from build123d import *

# Parameters (mm, degrees)
SKETCH_1_W               = 40
SKETCH_1_H               = 29
EXTRUDE_1_DEPTH          = 3
CUT_EXTRUDE_1_DEPTH      = 3
SKETCH_3_W               = 40
SKETCH_3_H               = 3
EXTRUDE_2_DEPTH          = 10
SKETCH_4_W               = 40
SKETCH_4_H               = 3
EXTRUDE_3_DEPTH          = 10
SKETCH_6_W               = 3
SKETCH_6_H               = 49
EXTRUDE_5_DEPTH          = 42
SKETCH_8_W               = 3
SKETCH_8_H               = 49
EXTRUDE_6_DEPTH          = 2
SKETCH_9_W               = 3
SKETCH_9_H               = 49
EXTRUDE_7_DEPTH          = 2
SKETCH_10_W              = 86
SKETCH_10_H              = 3
EXTRUDE_8_DEPTH          = 10
SKETCH_11_W              = 86
SKETCH_11_H              = 3
EXTRUDE_9_DEPTH          = 10
SKETCH_14_W              = 3
SKETCH_14_H              = 69
CUT_EXTRUDE_5_DEPTH      = 43
SKETCH_17_W              = 43
SKETCH_17_H              = 3
EXTRUDE_10_DEPTH         = 20
SKETCH_18_R              = 2.05
CUT_EXTRUDE_6_DEPTH      = 10
SKETCH_20_W              = 43
SKETCH_20_H              = 3
EXTRUDE_11_DEPTH         = 10
SKETCH_21_W              = 43
SKETCH_21_H              = 3
CUT_EXTRUDE_7_DEPTH      = 10
SKETCH_24_W              = 43
SKETCH_24_H              = 3
EXTRUDE_12_DEPTH         = 10
SKETCH_28_R              = 1.6
SKETCH_28_R_2            = 6.1
CUT_EXTRUDE_9_DEPTH      = 10
SKETCH_29_W              = 43
SKETCH_29_H              = 3
CUT_EXTRUDE_10_DEPTH     = 20
SKETCH_30_R              = 2.05
CUT_EXTRUDE_11_DEPTH     = 10
M3X0_5_1_D               = 2.5
M3X0_5_1_DEPTH           = 8.5
M3X0_5_1_TIP             = 0.751075774
M3X0_5_1_ON_FACE_2_D     = 2.5
M3X0_5_1_ON_FACE_2_DEPTH = 8.5
M3X0_5_1_ON_FACE_2_TIP   = 0.751075774
SKETCH_32_W              = 43
SKETCH_32_H              = 3
CUT_EXTRUDE_12_DEPTH     = 8


with BuildPart() as part:
    # ｽｹｯﾁ1 → ﾎﾞｽ - 押し出し1 (new body)
    with BuildSketch(Plane.XY):
        Rectangle(SKETCH_1_W, SKETCH_1_H)
    extrude(amount=EXTRUDE_1_DEPTH)

    # ｽｹｯﾁ2 → ｶｯﾄ - 押し出し1 (cut)
    with BuildSketch(Plane.XY.offset(3)):
        with BuildLine():
            ThreePointArc((-14.4, 10.5), (-15.01507576, 11.98492424), (-16.5, 12.6))
            Line((-16.5, 12.6), (-16.5, 10.5))
            Line((-16.5, 10.5), (-18.6, 10.5))
            ThreePointArc((-18.6, 10.5), (-16.5, 8.4), (-14.4, 10.5))
        make_face()
        with BuildLine():
            Line((-16.5, 10.5), (-16.5, 12.6))
            ThreePointArc((-16.5, 12.6), (-17.98492424, 11.98492424), (-18.6, 10.5))
            Line((-18.6, 10.5), (-16.5, 10.5))
        make_face()
        with BuildLine():
            ThreePointArc((-18.6, -10.5), (-17.98492424, -11.98492424), (-16.5, -12.6))
            Line((-16.5, -12.6), (-16.5, -10.5))
            Line((-16.5, -10.5), (-18.6, -10.5))
        make_face()
        with BuildLine():
            Line((-16.5, -10.5), (-16.5, -12.6))
            ThreePointArc((-16.5, -12.6), (-15.01507576, -11.98492424), (-14.4, -10.5))
            ThreePointArc((-14.4, -10.5), (-16.5, -8.4), (-18.6, -10.5))
            Line((-18.6, -10.5), (-16.5, -10.5))
        make_face()
        with BuildLine():
            ThreePointArc((18.6, -10.5), (15.01507576, -9.01507576), (16.5, -12.6))
            Line((16.5, -12.6), (16.5, -10.5))
            Line((16.5, -10.5), (18.6, -10.5))
        make_face()
        with BuildLine():
            Line((16.5, -10.5), (16.5, -12.6))
            ThreePointArc((16.5, -12.6), (17.98492424, -11.98492424), (18.6, -10.5))
            Line((18.6, -10.5), (16.5, -10.5))
        make_face()
        with BuildLine():
            ThreePointArc((18.6, 10.5), (17.98492424, 11.98492424), (16.5, 12.6))
            Line((16.5, 12.6), (16.5, 10.5))
            Line((16.5, 10.5), (18.6, 10.5))
        make_face()
        with BuildLine():
            Line((16.5, 10.5), (16.5, 12.6))
            ThreePointArc((16.5, 12.6), (15.01507576, 9.01507576), (18.6, 10.5))
            Line((18.6, 10.5), (16.5, 10.5))
        make_face()
    extrude(amount=-CUT_EXTRUDE_1_DEPTH, mode=Mode.SUBTRACT)

    # ｽｹｯﾁ3 → ﾎﾞｽ - 押し出し2 (add)
    with BuildSketch(Plane.XZ.offset(14.5)):
        with Locations((0, 1.5)):
            Rectangle(SKETCH_3_W, SKETCH_3_H)
    extrude(amount=EXTRUDE_2_DEPTH)

    # ｽｹｯﾁ4 → ﾎﾞｽ - 押し出し3 (add)
    with BuildSketch(Plane(origin=(0, 14.5, 0), x_dir=(1, 0, 0), z_dir=(0, 1, 0))):
        with Locations((0, -1.5)):
            Rectangle(SKETCH_4_W, SKETCH_4_H)
    extrude(amount=EXTRUDE_3_DEPTH)

    # ｽｹｯﾁ6 → ﾎﾞｽ - 押し出し5 (add)
    with BuildSketch(Plane(origin=(20, 0, 0), x_dir=(0, 0, -1), z_dir=(1, 0, 0))):
        with Locations((-1.5, 0)):
            Rectangle(SKETCH_6_W, SKETCH_6_H)
    extrude(amount=EXTRUDE_5_DEPTH)

    # ｽｹｯﾁ8 → ﾎﾞｽ - 押し出し6 (add)
    with BuildSketch(Plane.ZY.offset(20)):
        with Locations((1.5, 0)):
            Rectangle(SKETCH_8_W, SKETCH_8_H)
    extrude(amount=EXTRUDE_6_DEPTH)

    # ｽｹｯﾁ9 → ﾎﾞｽ - 押し出し7 (add)
    with BuildSketch(Plane(origin=(62, 0, 0), x_dir=(0, 0, -1), z_dir=(1, 0, 0))):
        with Locations((-1.5, 0)):
            Rectangle(SKETCH_9_W, SKETCH_9_H)
    extrude(amount=EXTRUDE_7_DEPTH)

    # ｽｹｯﾁ10 → ﾎﾞｽ - 押し出し8 (add)
    with BuildSketch(Plane.XZ.offset(24.5)):
        with Locations((21, 1.5)):
            Rectangle(SKETCH_10_W, SKETCH_10_H)
    extrude(amount=EXTRUDE_8_DEPTH)

    # ｽｹｯﾁ11 → ﾎﾞｽ - 押し出し9 (add)
    with BuildSketch(Plane(origin=(0, 24.5, 0), x_dir=(1, 0, 0), z_dir=(0, 1, 0))):
        with Locations((21, -1.5)):
            Rectangle(SKETCH_11_W, SKETCH_11_H)
    extrude(amount=EXTRUDE_9_DEPTH)

    # ｽｹｯﾁ14 → ｶｯﾄ - 押し出し5 (cut)
    with BuildSketch(Plane.ZY.offset(22)):
        with Locations((1.5, 0)):
            Rectangle(SKETCH_14_W, SKETCH_14_H)
    extrude(amount=-CUT_EXTRUDE_5_DEPTH, mode=Mode.SUBTRACT)

    # ｽｹｯﾁ17 → ﾎﾞｽ - 押し出し10 (add)
    with BuildSketch(Plane.XZ.offset(34.5)):
        with Locations((42.5, 1.5)):
            Rectangle(SKETCH_17_W, SKETCH_17_H)
    extrude(amount=EXTRUDE_10_DEPTH)

    # ｽｹｯﾁ18 → ｶｯﾄ - 押し出し6 (cut)
    with BuildSketch(Plane.XY.offset(3)):
        with Locations((28, -34.5)):
            Circle(SKETCH_18_R)
        with Locations((57, -34.5)):
            Circle(SKETCH_18_R)
    extrude(amount=-CUT_EXTRUDE_6_DEPTH, mode=Mode.SUBTRACT)

    # ｽｹｯﾁ20 → ﾎﾞｽ - 押し出し11 (add)
    with BuildSketch(Plane.XZ.offset(54.5)):
        with Locations((42.5, 1.5)):
            Rectangle(SKETCH_20_W, SKETCH_20_H)
    extrude(amount=EXTRUDE_11_DEPTH)

    # ｽｹｯﾁ21 → ｶｯﾄ - 押し出し7 (cut)
    with BuildSketch(Plane(origin=(0, 34.5, 0), x_dir=(1, 0, 0), z_dir=(0, 1, 0))):
        with Locations((42.5, -1.5)):
            Rectangle(SKETCH_21_W, SKETCH_21_H)
    extrude(amount=-CUT_EXTRUDE_7_DEPTH, mode=Mode.SUBTRACT)

    # ｽｹｯﾁ24 → ﾎﾞｽ - 押し出し12 (add)
    with BuildSketch(Plane(origin=(0, 24.5, 0), x_dir=(1, 0, 0), z_dir=(0, 1, 0))):
        with Locations((42.5, -1.5)):
            Rectangle(SKETCH_24_W, SKETCH_24_H)
    extrude(amount=EXTRUDE_12_DEPTH)

    # ｽｹｯﾁ28 → ｶｯﾄ - 押し出し9 (cut)
    with BuildSketch(Plane.XY.offset(3)):
        with Locations((42.5, 11.25)):
            Circle(SKETCH_28_R)
        with Locations((28.86009989, 3.375)):
            Circle(SKETCH_28_R)
        with Locations((56.13990011, 3.375)):
            Circle(SKETCH_28_R)
        with Locations((35.5, -4.5)):
            Circle(SKETCH_28_R_2)
        with Locations((56.13990011, -12.375)):
            Circle(SKETCH_28_R)
        with Locations((42.5, -20.25)):
            Circle(SKETCH_28_R)
        with Locations((28.86009989, -12.375)):
            Circle(SKETCH_28_R)
    extrude(amount=-CUT_EXTRUDE_9_DEPTH, mode=Mode.SUBTRACT)

    # ｽｹｯﾁ29 → ｶｯﾄ - 押し出し10 (cut)
    with BuildSketch(Plane(origin=(0, -64.5, 0), x_dir=(-1, 0, 0), z_dir=(0, -1, 0))):
        with Locations((-42.5, -1.5)):
            Rectangle(SKETCH_29_W, SKETCH_29_H)
    extrude(amount=-CUT_EXTRUDE_10_DEPTH, mode=Mode.SUBTRACT)

    # ｽｹｯﾁ30 → ｶｯﾄ - 押し出し11 (cut)
    with BuildSketch(Plane.XY.offset(3)):
        with Locations((42.5, -34.5)):
            Circle(SKETCH_30_R)
    extrude(amount=-CUT_EXTRUDE_11_DEPTH, mode=Mode.SUBTRACT)

    # M3x0.5 ねじ穴1
    with Locations(Plane(origin=(24, 13.5, 3), x_dir=(1, 0, 0), z_dir=(0, 0, 1))):
        with Locations((0, 0), (22.2, 10.3)):
            Hole(M3X0_5_1_D / 2, depth=M3X0_5_1_DEPTH)
            with Locations((0, 0, -(M3X0_5_1_DEPTH + M3X0_5_1_TIP / 2))):  # 118° drill point
                Cone(0, M3X0_5_1_D / 2, M3X0_5_1_TIP, mode=Mode.SUBTRACT)

    # M3x0.5 ねじ穴1 on face 2
    with Locations(Plane(origin=(29.171215171, -61.022508803, 0), x_dir=(1, 0, 0), z_dir=(0, 0, 1))):
        with Locations((0, 0)):
            Hole(M3X0_5_1_ON_FACE_2_D / 2, depth=M3X0_5_1_ON_FACE_2_DEPTH)
            with Locations((0, 0, -(M3X0_5_1_ON_FACE_2_DEPTH + M3X0_5_1_ON_FACE_2_TIP / 2))):  # 118° drill point
                Cone(0, M3X0_5_1_ON_FACE_2_D / 2, M3X0_5_1_ON_FACE_2_TIP, mode=Mode.SUBTRACT)

    # ｽｹｯﾁ32 → ｶｯﾄ - 押し出し12 (cut)
    with BuildSketch(Plane(origin=(0, 34.5, 0), x_dir=(1, 0, 0), z_dir=(0, 1, 0))):
        with Locations((42.5, -1.5)):
            Rectangle(SKETCH_32_W, SKETCH_32_H)
    extrude(amount=-CUT_EXTRUDE_12_DEPTH, mode=Mode.SUBTRACT)


solid = part.part
The listing builds one solid part. Answer for the finished solid, in the listing's coordinates (mm). Give positions to 0.01 mm unless a question says otherwise; leave off trailing zeros. Order: outer loops, then holes, each group sorted by start corner. A loop starts at its lowest first (then second) coordinate and runs counter-clockwise, first axis right, second up. Notation, with made-up numbers: (-3, -40) - (5, -40) arc R13 cw to (5, -22) - close; hole circle Ø9 at (-12, 38.5). An arc over 180 degrees is marked (long way). One line per item, written item: value. Start each with the question number.
1) The mould has two halves that part along X. Classify faces 1 (the face through (43, -44.5, 1)), 2 (the face through (64, -9, 2)), 3 (the face through (45.045, 23.321, 1.479)), 4 (the face through (54.54, 3.45, 1.52)): released by +X, released by -X, zero draft, split by the parting line, or undercut.
2) A cutting plane is placed at B-B on x = 46.2. Give the vertices of the cut face in (y, z), then the cut area to 4 significant figures.
3) A cutting plane is placed at A-A on y = -34.5. Give the vertices of the cut face in (x, z), then the cut area to 3 significant figures.
4) Given pin 1 Ø3 at (x, y) = (56.14, 3.38) entering from +Z, flat-ended and moving along its own axis, determine where the tip first touches the part or whether it passes through.
5) A cutting plane is placed at D-D on x = 28. Give the vertices of the cut face in (y, z).
6) Find the intervals of material crossed by L1, parallel to Y at x = 46.2, z = 1.4; L2, parallel to Y at x = 57.5, z = 1.5; L3, parallel to Y at x = 57, z = 1, in increasing order.
7) A cutting plane is placed at C-C on y = -20.25. Give the vertices of the cut face in (x, z).
Answer sheet:
1. face 1: zero draft
1. face 2: released by +X
1. face 3: undercut
1. face 4: undercut
2. outline: (-44.5, 0) - (22.55, 0) - (22.55, 3) - (-44.5, 3) - close; (25.05, 0) - (26.5, 0) - (26.5, 3) - (25.05, 3) - close
2. area: 205.5 mm2
3. outline: (21, 0) - (25.95, 0) - (25.95, 3) - (21, 3) - close; (30.05, 0) - (40.45, 0) - (40.45, 3) - (30.05, 3) - close; (44.55, 0) - (54.95, 0) - (54.95, 3) - (44.55, 3) - close; (59.05, 0) - (64, 0) - (64, 3) - (59.05, 3) - close
3. area: 92.1 mm2
4. pin 1: passes through
5. outline: (-44.5, 0) - (-36.55, 0) - (-36.55, 3) - (-44.5, 3) - close; (-32.45, 0) - (-13.72, 0) - (-13.72, 3) - (-32.45, 3) - close; (-11.03, 0) - (2.03, 0) - (2.03, 3) - (-11.03, 3) - close; (4.72, 0) - (26.5, 0) - (26.5, 3) - (4.72, 3) - close
6. L1: y = -44.5 to 22.55, 25.05 to 26.5
6. L2: y = -44.5 to -36.49, -32.51 to -13.22, -11.53 to 2.53, 4.22 to 26.5
6. L3: y = -44.5 to -36.55, -32.45 to -13.72, -11.03 to 2.03, 4.72 to 26.5
7. outline: (21, 0) - (40.9, 0) - (40.9, 3) - (21, 3) - close; (44.1, 0) - (64, 0) - (64, 3) - (44.1, 3) - close
